Verification items for the finished model (mm, model axes). A direction names the side the tool comes from. Coordinates: 2 decimals unless noted, no trailing zeros. Write each loop counter-clockwise with the first axis right and the second up, starting at its lowest first coordinate (ties: lowest second). Pieces come first, ordered by that corner, then holes. Notation, with made-up numbers: (85, 56.5) -> (136, 56.5) arc R29 ccw to (136, 86.5) -> close; hole circle Ø10 at (-5.5, -16). An arc over 180 degrees is marked (long way). Answer in a Markdown table with one row per item.
```python
from build123d import *

# Parameters (mm, degrees)
F1_DEPTH = 7.5
F2_T     = -2


with BuildPart() as f1:
    # F0 (on Top) → F1 (new body, symmetric)
    with BuildSketch(Plane.XY):
        with BuildLine():
            Line((-92.5, -77.5), (92.5, -77.5))
            ThreePointArc((92.5, -77.5), (99.571068, -74.571068), (102.5, -67.5))
            Line((102.5, -67.5), (102.5, 67.5))
            ThreePointArc((102.5, 67.5), (99.571068, 74.571068), (92.5, 77.5))
            Line((92.5, 77.5), (-92.5, 77.5))
            ThreePointArc((-92.5, 77.5), (-99.571068, 74.571068), (-102.5, 67.5))
            Line((-102.5, 67.5), (-102.5, -67.5))
            ThreePointArc((-102.5, -67.5), (-99.571068, -74.571068), (-92.5, -77.5))
        make_face()
    extrude(amount=F1_DEPTH, both=True)

    # F2
    f2_openings = [f1.faces().sort_by_distance(p)[0] for p in [
        (0, 0, -7.5),
    ]]
    offset(amount=F2_T, openings=f2_openings)


solid = f1.part
```
1. Section check B-B, the plane x = -68.5. Record the boundary of the cut face in (y, z).
Geometry says:
| item | result |
|---|---|
| outline | (-77.5, -7.5) -> (-75.5, -7.5) -> (-75.5, 5.5) -> (75.5, 5.5) -> (75.5, -7.5) -> (77.5, -7.5) -> (77.5, 7.5) -> (-77.5, 7.5) -> close |
2. Tool access check on faces 4 (the cylindrical face through (99.49, -74.65, 0.11)), 5 (the flat face through (1, 75.5, -1)). Record the directions out of +Z, -Z, +X, -X, +Y, -Y that give a thin tool (end or side, any length) a straight path to the whole face; none if there is none.
Geometry says:
| item | result |
|---|---|
| face 4 | +Z, -Z, +X, -Y |
| face 5 | -Z |
3. Thickness scan on line 1 (X direction, y = 42.5, z = -4.75); line 2 (Y direction, x = -16, z = -4.75); line 3 (Z direction, x = 34.5, y = -24.5). Record the ranges inside material, lowest first. Write a range as from..to.
Geometry says:
| item | result |
|---|---|
| line 1 | -102.5..-100.5, 100.5..102.5 |
| line 2 | -77.5..-75.5, 75.5..77.5 |
| line 3 | 5.5..7.5 |
4. Mould release check, pull along X, two halves, no side actions. Record for faces 1 (the flat face through (-1, 1, 5.5)), 2 (the flat face through (1, 77.5, 0)), 3 (the flat face through (102.5, -1, 0)): released by +X, released by -X, zero draft, split by the parting line, or undercut.
Geometry says:
| item | result |
|---|---|
| face 1 | undercut |
| face 2 | zero draft |
| face 3 | released by +X |
5. Section check A-A, the plane y = -17. Record the boundary of the cut face in (x, z), plus the area to 3 significant figures.
Geometry says:
| item | result |
|---|---|
| outline | (-102.5, -7.5) -> (-100.5, -7.5) -> (-100.5, 5.5) -> (100.5, 5.5) -> (100.5, -7.5) -> (102.5, -7.5) -> (102.5, 7.5) -> (-102.5, 7.5) -> close |
| area | 462 mm^2 |
6. Section check C-C, the plane z = 3. Record the boundary of the cut face in (x, y).
Geometry says:
| item | result |
|---|---|
| outline | (-102.5, -67.5) arc R10 ccw to (-92.5, -77.5) -> (92.5, -77.5) arc R10 ccw to (102.5, -67.5) -> (102.5, 67.5) arc R10 ccw to (92.5, 77.5) -> (-92.5, 77.5) arc R10 ccw to (-102.5, 67.5) -> close; hole (-100.5, -67.5) arc R8 ccw to (-92.5, -75.5) -> (92.5, -75.5) arc R8 ccw to (100.5, -67.5) -> (100.5, 67.5) arc R8 ccw to (92.5, 75.5) -> (-92.5, 75.5) arc R8 ccw to (-100.5, 67.5) -> close |
